Check sheet for the modelled part. Datum: model origin and axes. Units: mm. A direction names the side the tool comes from. Coordinates: 2 decimals unless noted, no trailing zeros. Loops run counter-clockwise (first coordinate to the right, second up) from the corner with the lowest first, then second, coordinate; pieces in that order, holes last. Notation, with made-up numbers: (-37, -9.5) -> (4, -9.5) arc R11 cw to (4, -5.5) -> close; hole circle Ø1 at (40, 31). An arc over 180 degrees is marked (long way). Use one line per item in the form item = value.
from build123d import *

# Parameters (mm, degrees)
F0_W     = 55
F0_H     = 70
F1_DEPTH = 10
F3_DEPTH = 25


with BuildPart() as f1:
    # F0 (on Top) → F1 (new body)
    with BuildSketch(Plane.XY):
        with Locations((-16.4421387017, 12.7911348291)):
            Rectangle(F0_W, F0_H)
    extrude(amount=-F1_DEPTH)

    # F2 (on face) → F3 (join)
    with BuildSketch(Plane.XY):
        with BuildLine():
            Line((-41.7943287017, 12.7911348291), (-29.7943287017, 12.7911348291))
            ThreePointArc((-29.7943287017, 12.7911348291), (-35.7943287017, 18.7911348291), (-41.7943287017, 12.7911348291))
        make_face()
        with BuildLine():
            ThreePointArc((-41.7943287017, 12.7911348291), (-35.7943287017, 6.7911348291), (-29.7943287017, 12.7911348291))
            Line((-29.7943287017, 12.7911348291), (-41.7943287017, 12.7911348291))
        make_face()
        with BuildLine():
            Line((-22.4421387017, 12.7911348291), (-10.4421387017, 12.7911348291))
            ThreePointArc((-10.4421387017, 12.7911348291), (-16.4421387017, 18.7911348291), (-22.4421387017, 12.7911348291))
        make_face()
        with BuildLine():
            ThreePointArc((-22.4421387017, 12.7911348291), (-16.4421387017, 6.7911348291), (-10.4421387017, 12.7911348291))
            Line((-10.4421387017, 12.7911348291), (-22.4421387017, 12.7911348291))
        make_face()
        with BuildLine():
            Line((-2.9411387017, 12.7911348291), (9.0588612983, 12.7911348291))
            ThreePointArc((9.0588612983, 12.7911348291), (3.0588612983, 18.7911348291), (-2.9411387017, 12.7911348291))
        make_face()
        with BuildLine():
            ThreePointArc((-2.9411387017, 12.7911348291), (3.0588612983, 6.7911348291), (9.0588612983, 12.7911348291))
            Line((9.0588612983, 12.7911348291), (-2.9411387017, 12.7911348291))
        make_face()
    extrude(amount=F3_DEPTH)


solid = f1.part
(1) Scan lines: line 1 along X through (y, z) = (13.5, 3.5); line 2 along Z through (x, y) = (-16.5, -2); line 3 along X through (y, z) = (8, 12.5). Record each from-to range of solid material in increasing order.
Established:
line_1 = -41.75 to -29.84, -22.4 to -10.48, -2.9 to 9.02
line_2 = -10 to 0
line_3 = -39.41 to -32.18, -20.05 to -12.83, -0.55 to 6.67
(2) Section check C-C, the plane y = 36.5. Record the boundary of the cut face in (x, z), plus the area to 3 significant figures.
Established:
outline = (-43.94, -10) -> (11.06, -10) -> (11.06, 0) -> (-43.94, 0) -> close
area = 550 mm²
(3) Section check D-D, the plane x = -0.5. Record the boundary of the cut face in (y, z).
Established:
outline = (-22.21, -10) -> (47.79, -10) -> (47.79, 0) -> (17.62, 0) -> (17.62, 25) -> (7.96, 25) -> (7.96, 0) -> (-22.21, 0) -> close
(4) Tool access check on faces 5 (the cylindrical face through (-11.68, 16.44, 12.32)), 6 (the flat face through (-17, 13, 25)). Record the directions out of +Z, -Z, +X, -X, +Y, -Y that give a thin tool (end or side, any length) a straight path to the whole face; none if there is none.
Established:
face_5 = +Z
face_6 = +Z, +X, -X, +Y, -Y
(5) Section check A-A, the plane x = -33. Record the boundary of the cut face in (y, z), plus the area to 3 significant figures.
Established:
outline = (-22.21, -10) -> (47.79, -10) -> (47.79, 0) -> (18.1, 0) -> (18.1, 25) -> (7.48, 25) -> (7.48, 0) -> (-22.21, 0) -> close
area = 965 mm²
(6) Go/stop test with flat-tipped pins: P1, Ø2, axis at x = 5, z = 14, coming from the -Y side; P2, Ø1, axis at x = -31.5, z = 8.5, coming from the -Y side; P3, Ø12, axis at x = -35, z = 18, coming from the +Y side. Record where each tip stops, or that it passes through.
Established:
P1 = 6.87
P2 = 8.14
P3 = 18.79
(7) Section check B-B, the plane z = 3. Record the boundary of the cut face in (x, y).
Established:
outline = circle Ø12 at (-35.79, 12.79); circle Ø12 at (-16.44, 12.79); circle Ø12 at (3.06, 12.79)
(8) Mould release check, pull along X, two halves, no side actions. Record for faces 1 (the cylindrical face through (4.36, 18.65, 12.32)), 2 (the flat face through (-43.942, 12, -5)), 3 (the cylindrical face through (-41.337, 15.089, 12.325)), 4 (the flat face through (3, 13, 25)): +X half, -X half, draft (parallel to the pull), parting line (faces both ways), or undercut.
Established:
face_1 = undercut
face_2 = -X half
face_3 = undercut
face_4 = draft
